from build123d import *

# Parameters (mm, degrees)
SKETCH020_R           = 3.5
POCKET008_DEPTH       = 100
POCKET008_DEPTH_BACK  = 100
POLARPATTERN005_COUNT = 30
SKETCH021_R           = 3
POCKET009_DEPTH       = 100
POCKET009_DEPTH_BACK  = 100
POLARPATTERN006_COUNT = 25
SKETCH022_R           = 2.5
POCKET010_DEPTH       = 100
POCKET010_DEPTH_BACK  = 100
POLARPATTERN007_COUNT = 20
SKETCH023_R           = 2
POCKET011_DEPTH       = 100
POCKET011_DEPTH_BACK  = 100
POLARPATTERN008_COUNT = 15
SKETCH024_R           = 1.5
POCKET012_DEPTH       = 100
POCKET012_DEPTH_BACK  = 100
POLARPATTERN009_COUNT = 10
SKETCH025_R           = 3
POCKET013_DEPTH       = 100
POCKET013_DEPTH_BACK  = 100


with BuildPart() as part:
    # Sketch019 → Revolution003 (revolve)
    with BuildSketch(Plane.XZ):
        Polygon((-55, -20), (0, -20), (0, -26), (-51, -26), (-51, -23), (-55, -23), align=None)
    revolve(axis=Axis((0, 0, 0), (0, 0, 1)))

    # Sketch020 → Pocket008 (cut, two sides)
    with BuildSketch(Plane.XY) as pocket008_sk:
        with Locations((-46, 0)):
            Circle(SKETCH020_R)
    pocket008 = extrude(amount=-POCKET008_DEPTH, mode=Mode.SUBTRACT) + extrude(pocket008_sk.sketch, amount=POCKET008_DEPTH_BACK, mode=Mode.SUBTRACT)

    # PolarPattern005: Pocket008 ×30 about axis
    polarpattern005_axis = Axis((0, 0, 0), (0, 0, 1))
    for i in range(1, POLARPATTERN005_COUNT):
        add(pocket008.rotate(polarpattern005_axis, i * 360 / POLARPATTERN005_COUNT), mode=Mode.SUBTRACT)

    # Sketch021 → Pocket009 (cut, two sides)
    with BuildSketch(Plane.XY) as pocket009_sk:
        with Locations((-36, 0)):
            Circle(SKETCH021_R)
    pocket009 = extrude(amount=-POCKET009_DEPTH, mode=Mode.SUBTRACT) + extrude(pocket009_sk.sketch, amount=POCKET009_DEPTH_BACK, mode=Mode.SUBTRACT)

    # PolarPattern006: Pocket009 ×25 about axis
    polarpattern006_axis = Axis((0, 0, 0), (0, 0, 1))
    for i in range(1, POLARPATTERN006_COUNT):
        add(pocket009.rotate(polarpattern006_axis, i * 360 / POLARPATTERN006_COUNT), mode=Mode.SUBTRACT)

    # Sketch022 → Pocket010 (cut, two sides)
    with BuildSketch(Plane.XY) as pocket010_sk:
        with Locations((-26, 0)):
            Circle(SKETCH022_R)
    pocket010 = extrude(amount=-POCKET010_DEPTH, mode=Mode.SUBTRACT) + extrude(pocket010_sk.sketch, amount=POCKET010_DEPTH_BACK, mode=Mode.SUBTRACT)

    # PolarPattern007: Pocket010 ×20 about axis
    polarpattern007_axis = Axis((0, 0, 0), (0, 0, 1))
    for i in range(1, POLARPATTERN007_COUNT):
        add(pocket010.rotate(polarpattern007_axis, i * 360 / POLARPATTERN007_COUNT), mode=Mode.SUBTRACT)

    # Sketch023 → Pocket011 (cut, two sides)
    with BuildSketch(Plane.XY) as pocket011_sk:
        with Locations((-16, 0)):
            Circle(SKETCH023_R)
    pocket011 = extrude(amount=-POCKET011_DEPTH, mode=Mode.SUBTRACT) + extrude(pocket011_sk.sketch, amount=POCKET011_DEPTH_BACK, mode=Mode.SUBTRACT)

    # PolarPattern008: Pocket011 ×15 about axis
    polarpattern008_axis = Axis((0, 0, 0), (0, 0, 1))
    for i in range(1, POLARPATTERN008_COUNT):
        add(pocket011.rotate(polarpattern008_axis, i * 360 / POLARPATTERN008_COUNT), mode=Mode.SUBTRACT)

    # Sketch024 → Pocket012 (cut, two sides)
    with BuildSketch(Plane.XY) as pocket012_sk:
        with Locations((-8, 0)):
            Circle(SKETCH024_R)
    pocket012 = extrude(amount=-POCKET012_DEPTH, mode=Mode.SUBTRACT) + extrude(pocket012_sk.sketch, amount=POCKET012_DEPTH_BACK, mode=Mode.SUBTRACT)

    # PolarPattern009: Pocket012 ×10 about axis
    polarpattern009_axis = Axis((0, 0, 0), (0, 0, 1))
    for i in range(1, POLARPATTERN009_COUNT):
        add(pocket012.rotate(polarpattern009_axis, i * 360 / POLARPATTERN009_COUNT), mode=Mode.SUBTRACT)

    # Sketch025 → Pocket013 (cut, two sides)
    with BuildSketch(Plane.XY) as pocket013_sk:
        Circle(SKETCH025_R)
    extrude(amount=-POCKET013_DEPTH, mode=Mode.SUBTRACT)
    extrude(pocket013_sk.sketch, amount=POCKET013_DEPTH_BACK, mode=Mode.SUBTRACT)


solid = part.part
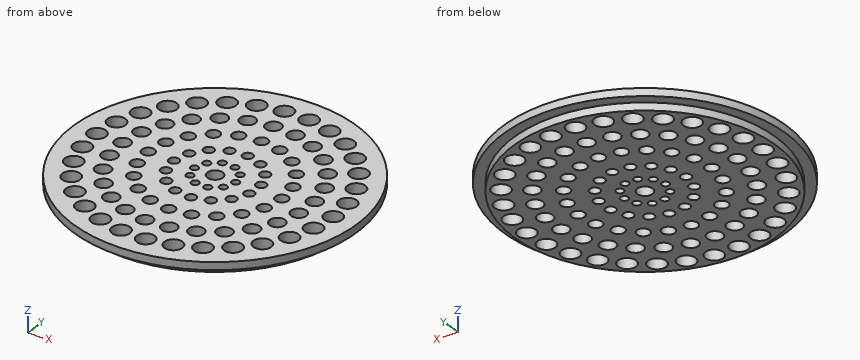
Geometry: final body of the model. Coordinates: model frame, mm. Coordinates: 2 decimals unless noted, no trailing zeros.
1) Section A-A (z = -24.45). Give the number of separate pieces and of enclosed holes in the cut face, then the cut area to 3 significant figures.
Result sheet:
separate pieces: 1
enclosed holes: 101
area: 5,630 mm2
2) First-contact query: P1, Ø11, axis at x = 4.81, y = 45.75, coming from the -Z side; P2, Ø3, axis at x = -16, y = 0, coming from the -Z side; P3, Ø1.5, axis at y = -18.5, z = -21, coming from the +X side; P4, Ø1, axis at y = -3.5, z = -24.5, coming from the +X side. Flat tips, straight axial feed; report the tip coordinate or a pass-through.
Result sheet:
P1: stops at z = -26
P2: passes through
P3: stops at x = 52.06
P4: stops at x = 50.91
3) Ray query, probe 1 along Y at (x, z) = (26, -22.15); probe 2 along Y at (x, z) = (30, -23.15); probe 3 along X at (y, z) = (46, -22.3) (3 decimals). Return the intervals inside material, ascending.
Result sheet:
probe 1: y = -48.47 to -41.64, -38.03 to -10.19, -5.88 to -2.5, 2.5 to 5.88, 10.19 to 38.03, 41.64 to 48.47
probe 2: y = -41.24 to -37.6, -30.77 to -24.03, -18.29 to 18.29, 24.03 to 30.77, 37.6 to 41.24
probe 3: x = -30.15 to -16.895, -11.535 to -8.299, -1.317 to 1.317, 8.299 to 11.535, 16.895 to 30.15
